```python
from build123d import *

# Parameters (mm, degrees)
TAGLIO_ESTRUSIONE3_START = -1.5
TAGLIO_ESTRUSIONE3_DEPTH = 1.5


# Read off the part's stored shape, not the designer's step: Taglio-Estrusione3
with BuildPart() as part:
    # Schizzo2 → Rivoluzione2 (revolve)
    with BuildSketch(Plane.XY):
        with BuildLine():
            ThreePointArc((3, 0), (1.677059909, -1.104119819), (0, -1.5))
            Line((0, -1.5), (0, 0))
            Line((0, 0), (3, 0))
        make_face()
    revolve(axis=Axis((0, -1.5, 0), (0, 1, 0)))

    # Taglio-Estrusione3 outline → Taglio-Estrusione3 (cut)
    with BuildSketch(Plane(origin=(0, -1.5, 0), x_dir=(-1, 0, 0), z_dir=(0, -1, 0)).offset(TAGLIO_ESTRUSIONE3_START)):
        with BuildLine():
            Line((0.1, 2.096662955), (-0.1, 2.096662955))
            Line((-0.1, 2.096662955), (-0.1, 1.496662955))
            ThreePointArc((-0.1, 1.496662955), (-0.881677879, 1.213525492), (-1.392509356, 0.557599939))
            Line((-1.392509356, 0.557599939), (-1.98100003, 0.74881215))
            Line((-1.98100003, 0.74881215), (-2.042803429, 0.558600847))
            Line((-2.042803429, 0.558600847), (-1.454312755, 0.367388636))
            ThreePointArc((-1.454312755, 0.367388636), (-1.426584774, -0.463525492), (-0.960618112, -1.15204724))
            Line((-0.960618112, -1.15204724), (-1.309372877, -1.632066993))
            Line((-1.309372877, -1.632066993), (-1.147569478, -1.749624043))
            Line((-1.147569478, -1.749624043), (-0.798814713, -1.26960429))
            ThreePointArc((-0.798814713, -1.26960429), (0, -1.5), (0.798814713, -1.26960429))
            Line((0.798814713, -1.26960429), (1.147569478, -1.749624043))
            Line((1.147569478, -1.749624043), (1.309372877, -1.632066993))
            Line((1.309372877, -1.632066993), (0.960618112, -1.15204724))
            ThreePointArc((0.960618112, -1.15204724), (1.426584774, -0.463525492), (1.454312755, 0.367388636))
            Line((1.454312755, 0.367388636), (2.024738008, 0.552731036))
            Line((2.024738008, 0.552731036), (1.962934609, 0.742942339))
            Line((1.962934609, 0.742942339), (1.392509356, 0.557599939))
            ThreePointArc((1.392509356, 0.557599939), (0.881677879, 1.213525492), (0.1, 1.496662955))
            Line((0.1, 1.496662955), (0.1, 2.096662955))
        make_face()
    extrude(amount=TAGLIO_ESTRUSIONE3_DEPTH, mode=Mode.SUBTRACT)


solid = part.part
```
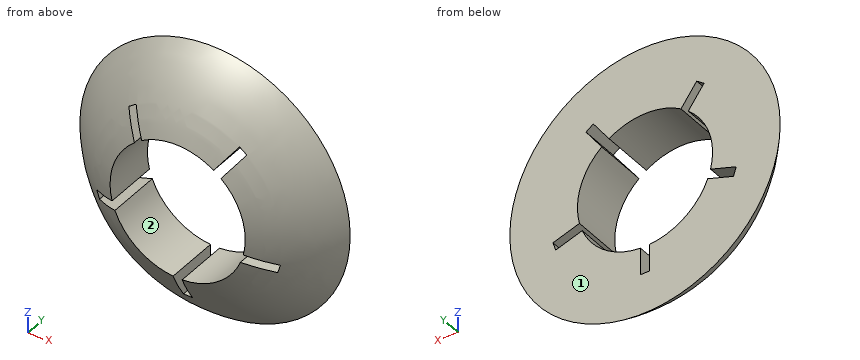
Could you check a few things on this model? Use its own coordinates, in mm. Face numbers are marked on the shaded views. Coordinates: 2 decimals unless noted, no trailing zeros. Write item = value, one per line. Start each with the question number.
(1) We'd pull the mould along X, two halves only. Please class the marked faces 1 and 2: released by +X, released by -X, zero draft, split by the parting line, or undercut.
(2) I want a section at A-A (y = -1). Give the number of separate pieces and of enclosed holes in the cut face, plus the area to 3 significant figures.
(3) I need wall thicknesses on line 1 (Z direction, x = -0.5, y = -0.8); line 2 (X direction, y = -0.8, z = 0.75); line 3 (X direction, y = -0.05, z = -1). Which ranges of each line are inside material? Lowest first, please. Write a range as [from, to].
Result set:
q1.face_1 = zero draft
q1.face_2 = undercut
q2.separate_pieces = 5
q2.enclosed_holes = 0
q2.area = 3.56 mm2
q3.line_1 = [-2.12, -1.41], [1.41, 2.12]
q3.line_2 = [-2.05, -1.3], [1.3, 2.05]
q3.line_3 = [-2.79, -1.12], [1.12, 2.79]
